from build123d import *

# Parameters (mm, degrees)
F1_DEPTH = 17.1
F0_W     = 31
F0_H     = 31
F0_R     = 9
F0_W_2   = 20.5
F2_DEPTH = 2
F3_DEPTH = 10
F4_R     = 15
F5_W     = 15.5
F5_H     = 5
F5_H_2   = 18.6
F6_DEPTH = 2
F7_D     = 3
F8_R     = 5


with BuildPart() as f1:
    # F0 (on Top) → F1 (new body)
    with BuildSketch(Plane.XY):
        Polygon((36, -15.5), (15.5, -15.5), (-15.5, -15.5), (-15.5, -34.1), (36, -34.1), align=None)
    extrude(amount=F1_DEPTH)

    # F0 (on Top) → F2 (join)
    with BuildSketch(Plane.XY):
        Rectangle(F0_W, F0_H)
        Circle(F0_R, mode=Mode.SUBTRACT)
        with Locations((25.75, 0)):
            Rectangle(F0_W_2, F0_H)
    extrude(amount=F2_DEPTH)

    # F0 (on Top) → F3 (join)
    with BuildSketch(Plane.XY):
        Polygon((-15.5, 15.5), (15.5, 15.5), (36, 15.5), (36, 17), (-15.5, 17), align=None)
    extrude(amount=F3_DEPTH)

    # F4
    f4_edges = [f1.edges().sort_by_distance(p)[0] for p in [
        (-15.5, 17, 5),
    ]]
    fillet(f4_edges, radius=F4_R)

    # F5 (on face) → F6 (join)
    with BuildSketch(Plane.XY.offset(17.1)):
        with Locations((28.25, -13)):
            Rectangle(F5_W, F5_H)
        with Locations((28.25, -24.8)):
            Rectangle(F5_W, F5_H_2)
    extrude(amount=F6_DEPTH)

    # F7 (through all)
    with Locations(Plane.XY.offset(17.1)):
        with Locations((0, -23.2)):
            Hole(F7_D / 2)

    # F8
    f8_edges = [f1.edges().sort_by_distance(p)[0] for p in [
        (-15.5, -15.5, 9.55),
    ]]
    fillet(f8_edges, radius=F8_R)


with BuildPart() as f9_1:
    # F9: instance of F1
    add(f1.part.mirror(Plane(origin=(36, -19.66422, 8.390388), x_dir=(0, 1, 0), z_dir=(1, 0, 0))))


solid = f9_1.part
Geometry: final body of the model. Coordinates: model frame, mm. A direction names the side the tool comes from. Give positions to 0.01 mm unless a question says otherwise; leave off trailing zeros. Write each loop counter-clockwise with the first axis right and the second up, starting at its lowest first coordinate (ties: lowest second). Pieces come first, ordered by that corner, then holes. Notation, with made-up numbers: (0.5, -33) -> (33.5, -33) arc R8 ccw to (33.5, -21) -> close; hole circle Ø10 at (9.5, 0.5). An arc over 180 degrees is marked (long way). Answer as a JSON object with one key per item and string values.
1. Cut plane B-B on y = 0. Output: boundary loops of the cut face in (x, z).
Ans:
{"outline": "(36, 0) -> (63, 0) -> (63, 2) -> (36, 2) -> close; (81, 0) -> (87.5, 0) -> (87.5, 2) -> (81, 2) -> close"}
2. Cut plane D-D on x = 67. Output: boundary loops of the cut face in (y, z), and give its area (3 significant figures).
Ans:
{"outline": "(-34.1, 0) -> (-7.48, 0) -> (-7.48, 2) -> (-15.5, 2) -> (-15.5, 17.1) -> (-34.1, 17.1) -> close; (7.48, 0) -> (17, 0) -> (17, 10) -> (15.5, 10) -> (15.5, 2) -> (7.48, 2) -> close", "area": "365 mm^2"}
3. Contact query for flat-ended pins moving along their axis: pin 1 (0.6 mm diameter, centred on x = 40.5, z = 17.5, fed in from +Y); pin 2 (1 mm diameter, centred on x = 56.5, y = -4, fed in from +Z); pin 3 (5 mm diameter, centred on x = 68.5, y = -23, fed in from -Z); pin 4 (0.6 mm diameter, centred on y = -25, z = 17.5, fed in from +X). Output: stop coordinate, or through.
Ans:
{"pin 1": "stops at y = -10.5", "pin 2": "stops at z = 2", "pin 3": "stops at z = 0", "pin 4": "stops at x = 51.5"}
4. Mould query, pull axis Y, two halves, no side actions, for faces 5 (the flat face through (44, -13, 17.1)), 6 (the flat face through (62, -2, 2)), 7 (the flat face through (54, 17, 5)). Classes: pulls with the +Y half, pulls with the -Y half, needs draft (parallel to the pull), parting line crosses it, or undercut.
Ans:
{"face 5": "needs draft", "face 6": "undercut", "face 7": "pulls with the +Y half"}
5. Cut plane A-A on z = 6.25. Output: boundary loops of the cut face in (x, y).
Ans:
{"outline": "(36, -34.1) -> (87.5, -34.1) -> (87.5, -20.5) arc R5 ccw to (82.5, -15.5) -> (36, -15.5) -> close; (36, 15.5) -> (79.04, 15.5) arc R15 ccw to (72.5, 17) -> (36, 17) -> close; hole circle Ø3 at (72, -23.2)"}
6. Cut plane C-C on z = 11.25. Output: boundary loops of the cut face in (x, y), and give its area (3 significant figures).
Ans:
{"outline": "(36, -34.1) -> (87.5, -34.1) -> (87.5, -20.5) arc R5 ccw to (82.5, -15.5) -> (36, -15.5) -> close; hole circle Ø3 at (72, -23.2)", "area": "945 mm^2"}
7. Ray query, probe 1 along Y at (x, z) = (72, 7.25); probe 2 along Y at (x, z) = (72, 1.6); probe 3 along Y at (x, z) = (51, 6). Return the intervals inside material, ascending. Write a range as from..to.
Ans:
{"probe 1": "y = -34.1..-24.7, -21.7..-15.5, 15.5..17", "probe 2": "y = -34.1..-24.7, -21.7..-9, 9..17", "probe 3": "y = -34.1..-15.5, 15.5..17"}
8. Access query for faces 1 (the flat face through (59, -15.5, 9)), 2 (the flat face through (58, 15.5, 6)), 3 (the flat face through (44, -10.5, 18)), 4 (the flat face through (70, -25, 17.1)). Directions: +Z, -Z, +X, -X, +Y, -Y. A direction counts if a zero-diameter tool reaches every point of the face in a straight line with its end or side. Return the directions, or none.
Ans:
{"face 1": "+X, -X", "face 2": "+Z, +X, -X", "face 3": "+Z, +X, -X, +Y", "face 4": "+Z, +X, +Y, -Y"}
